from build123d import *

# Parameters (mm, degrees)
SKETCH1_W           = 22
SKETCH1_H           = 13
BOSS_EXTRUDE1_DEPTH = 6
BOSS_EXTRUDE2_DEPTH = 2
BOSS_EXTRUDE3_DEPTH = 8
SKETCH4_R           = 1.525
SKETCH4_R_2         = 1.524
CUT_EXTRUDE1_DEPTH  = 36.566838488
SKETCH5_W           = 9
SKETCH5_H           = 4.088652256
CUT_EXTRUDE2_DEPTH  = 38.735924528
FILLET1_R           = 2
SKETCH6_W           = 12
SKETCH6_H           = 13.009000019
SKETCH6_W_2         = 15.838286437
CUT_EXTRUDE3_DEPTH  = 4
SKETCH7_W           = 2.5
SKETCH7_H           = 8
BOSS_EXTRUDE5_DEPTH = 3
FILLET3_R           = 2.5
FILLET4_R           = 2.5
SKETCH9_W           = 24
SKETCH9_H           = 8
CUT_EXTRUDE5_DEPTH  = 3
BOSS_EXTRUDE6_REACH = 35.526
SKETCH10_W          = 5
SKETCH10_H          = 2.5
BOSS_EXTRUDE7_DEPTH = 2
SKETCH12_R          = 7.5
BOSS_EXTRUDE8_DEPTH = 8
SKETCH13_R          = 3.8735
CUT_EXTRUDE6_DEPTH  = 8
FILLET5_R           = 1.5
FILLET7_R           = 1


with BuildPart() as part:
    # Sketch1 → Boss-Extrude1 (new body)
    with BuildSketch(Plane(origin=(0, 0, 0), x_dir=(1, 0, 0), z_dir=(0, 1, 0))):
        with BuildLine():
            Line((-1, -3), (23, -3))
            Line((23, -3), (25, -3))
            Line((25, -3), (25, -1))
            Line((25, -1), (25, 14))
            Line((25, 14), (25, 16))
            Line((25, 16), (23, 16))
            Line((23, 16), (-1, 16))
            ThreePointArc((-1, 16), (-2.414213562, 15.414213562), (-3, 14))
            Line((-3, 14), (-3, -1))
            ThreePointArc((-3, -1), (-2.414213562, -2.414213562), (-1, -3))
        make_face()
        with Locations((11, 6.5)):
            Rectangle(SKETCH1_W, SKETCH1_H, mode=Mode.SUBTRACT)
    extrude(amount=BOSS_EXTRUDE1_DEPTH)

    # Sketch2 → Boss-Extrude2 (add)
    with BuildSketch(Plane(origin=(0, 6, 0), x_dir=(1, 0, 0), z_dir=(0, 1, 0))):
        with BuildLine():
            Line((25, 14), (25, -1))
            Line((25, -1), (25, -3))
            Line((25, -3), (23, -3))
            Line((23, -3), (-1, -3))
            ThreePointArc((-1, -3), (-2.414213562, -2.414213562), (-3, -1))
            Line((-3, -1), (-3, 14))
            ThreePointArc((-3, 14), (-2.414213562, 15.414213562), (-1, 16))
            Line((-1, 16), (23, 16))
            Line((23, 16), (25, 16))
            Line((25, 16), (25, 14))
        make_face()
    extrude(amount=BOSS_EXTRUDE2_DEPTH)

    # Sketch3 → Boss-Extrude3 (add)
    with BuildSketch(Plane.XZ):
        with BuildLine():
            Line((5, 3), (17, 3))
            Line((17, 3), (17, 5.5))
            ThreePointArc((17, 5.5), (15.389087297, 9.389087297), (11.5, 11))
            Line((11.5, 11), (10.5, 11))
            ThreePointArc((10.5, 11), (6.610912703, 9.389087297), (5, 5.5))
            Line((5, 5.5), (5, 3))
        make_face()
        with BuildLine():
            Line((17, -16), (5, -16))
            Line((5, -16), (5, -18.5))
            ThreePointArc((5, -18.5), (6.610912703, -22.389087297), (10.5, -24))
            Line((10.5, -24), (11.5, -24))
            ThreePointArc((11.5, -24), (15.389087297, -22.389087297), (17, -18.5))
            Line((17, -18.5), (17, -16))
        make_face()
    extrude(amount=-BOSS_EXTRUDE3_DEPTH)

    # Sketch4 → Cut-Extrude1 (cut, through all)
    with BuildSketch(Plane(origin=(0, 0, 0), x_dir=(-1, 0, 0), z_dir=(0, -1, 0))):
        with Locations(Location((-11, 20, 0), (0, 0, 90))):
            Circle(SKETCH4_R)
        with Locations(Location((-11, -7, 0), (0, 0, 90))):
            Circle(SKETCH4_R_2)
    extrude(amount=-CUT_EXTRUDE1_DEPTH, mode=Mode.SUBTRACT)

    # Sketch5 → Cut-Extrude2 (cut, through all)
    with BuildSketch(Plane(origin=(25, 0, 0), x_dir=(0, 0, -1), z_dir=(1, 0, 0))):
        with Locations((6.5, 2.044326128)):
            Rectangle(SKETCH5_W, SKETCH5_H)
    extrude(amount=-CUT_EXTRUDE2_DEPTH, mode=Mode.SUBTRACT)

    # Fillet1
    fillet1_edges = [part.edges().sort_by_distance(p)[0] for p in [
        (-1.5, 4.088652256, -11),
        (-1.5, 4.088652256, -2),
        (23.5, 4.088652256, -11),
        (23.5, 4.088652256, -2),
    ]]
    fillet(fillet1_edges, radius=FILLET1_R)

    # Sketch6 → Cut-Extrude3 (cut)
    with BuildSketch(Plane(origin=(0, 8, 0), x_dir=(1, 0, 0), z_dir=(0, 1, 0))):
        with Locations((11, 22.504500009)):
            Rectangle(SKETCH6_W, SKETCH6_H)
        with Locations((11.149066226, -9.50450001)):
            Rectangle(SKETCH6_W_2, SKETCH6_H)
    extrude(amount=-CUT_EXTRUDE3_DEPTH, mode=Mode.SUBTRACT)

    # Sketch7 → Boss-Extrude5 (add)
    with BuildSketch(Plane(origin=(25, 0, 0), x_dir=(0, 0, -1), z_dir=(1, 0, 0))):
        with Locations((17.25, 4)):
            Rectangle(SKETCH7_W, SKETCH7_H)
        with Locations((-4.25, 4)):
            Rectangle(SKETCH7_W, SKETCH7_H)
    extrude(amount=-BOSS_EXTRUDE5_DEPTH)

    # Fillet3
    fillet3_edges = [part.edges().sort_by_distance(p)[0] for p in [
        (22, 4, -16),
    ]]
    fillet(fillet3_edges, radius=FILLET3_R - 0.0001)  # a hair under: the kernel refuses the full size

    # Fillet4
    fillet4_edges = [part.edges().sort_by_distance(p)[0] for p in [
        (22, 4, 3),
    ]]
    fillet(fillet4_edges, radius=FILLET4_R - 0.0001)  # a hair under: the kernel refuses the full size

    # Sketch9 → Cut-Extrude5 (cut)
    with BuildSketch(Plane(origin=(25, 0, 0), x_dir=(0, 0, -1), z_dir=(1, 0, 0))):
        with Locations((6.5, 4)):
            Rectangle(SKETCH9_W, SKETCH9_H)
    extrude(amount=-CUT_EXTRUDE5_DEPTH, mode=Mode.SUBTRACT)

    # Boss-Extrude6: up to this face of the body (flat: up to its plane)
    boss_extrude6_end = Plane(part.part.faces().sort_by_distance((9.97036164, 0, 3.836684907))[0])
    # Sketch10 → Boss-Extrude6 (add, up to the picked face)
    with BuildSketch(Plane(origin=(0, 8, 0), x_dir=(1, 0, 0), z_dir=(0, 1, 0)), mode=Mode.PRIVATE) as boss_extrude6_sk1:
        with Locations((19.5, 17.25)):
            Rectangle(SKETCH10_W, SKETCH10_H)
    boss_extrude6_tool1 = split(extrude(boss_extrude6_sk1.sketch, amount=-BOSS_EXTRUDE6_REACH, mode=Mode.PRIVATE), bisect_by=boss_extrude6_end, keep=Keep.BOTH, mode=Mode.PRIVATE)
    # Sketch10 → Boss-Extrude6 (add, up to the picked face)
    with BuildSketch(Plane(origin=(0, 8, 0), x_dir=(1, 0, 0), z_dir=(0, 1, 0)), mode=Mode.PRIVATE) as boss_extrude6_sk2:
        with Locations((19.5, -4.25)):
            Rectangle(SKETCH10_W, SKETCH10_H)
    boss_extrude6_tool2 = split(extrude(boss_extrude6_sk2.sketch, amount=-BOSS_EXTRUDE6_REACH, mode=Mode.PRIVATE), bisect_by=boss_extrude6_end, keep=Keep.BOTH, mode=Mode.PRIVATE)
    add(boss_extrude6_tool1.solids().sort_by(Axis((19.5, 8, -17.25), (0, -1, 0)))[0])
    add(boss_extrude6_tool2.solids().sort_by(Axis((19.5, 8, 4.25), (0, -1, 0)))[0])

    # Sketch11 → Boss-Extrude7 (add)
    with BuildSketch(Plane(origin=(0, 8, 0), x_dir=(1, 0, 0), z_dir=(0, 1, 0))):
        with BuildLine():
            Line((17, -3), (-1, -3))
            ThreePointArc((-1, -3), (-2.414213562, -2.414213562), (-3, -1))
            Line((-3, -1), (-3, 14))
            ThreePointArc((-3, 14), (-2.414213562, 15.414213562), (-1, 16))
            Line((-1, 16), (17, 16))
            Line((17, 16), (17, 18.5))
            Line((17, 18.5), (22, 18.5))
            Line((22, 18.5), (22, -5.5))
            Line((22, -5.5), (17, -5.5))
            Line((17, -5.5), (17, -3))
        make_face()
    extrude(amount=BOSS_EXTRUDE7_DEPTH)

    # Sketch12 → Boss-Extrude8 (add)
    with BuildSketch(Plane(origin=(0, 10, 0), x_dir=(1, 0, 0), z_dir=(0, 1, 0))):
        with Locations(Location((9.5, 6.5, 0), (0, 0, 90))):
            Circle(SKETCH12_R)
    extrude(amount=BOSS_EXTRUDE8_DEPTH)

    # Sketch13 → Cut-Extrude6 (cut)
    with BuildSketch(Plane(origin=(0, 18, 0), x_dir=(1, 0, 0), z_dir=(0, 1, 0))):
        with Locations(Location((9.5, 6.5, 0), (0, 0, 270))):
            Circle(SKETCH13_R)
    extrude(amount=-CUT_EXTRUDE6_DEPTH, mode=Mode.SUBTRACT)

    # Fillet5
    fillet5_edges = [part.edges().sort_by_distance(p)[0] for p in [
        (9.5, 10, 1),
    ]]
    fillet(fillet5_edges, radius=FILLET5_R)

    # Fillet7
    fillet7_edges = [part.edges().sort_by_distance(p)[0] for p in [
        (9.5, 18, 1),
    ]]
    fillet(fillet7_edges, radius=FILLET7_R)


solid = part.part
Here's how the part is built. I have some questions about the finished solid (model axes, mm). A direction names the side the tool comes from. Round coordinates to 2 decimals unless told otherwise and drop trailing zeros. Write each loop counter-clockwise with the first axis right and the second up, starting at its lowest first coordinate (ties: lowest second). Pieces come first, ordered by that corner, then holes. Notation, with made-up numbers: (41.5, 42) -> (89.5, 42) arc R9 ccw to (89.5, 57) -> close; hole circle Ø10 at (-0.75, 12). An arc over 180 degrees is marked (long way). One line per item, written item: value.
1) Suppose I cut it at D-D on x = -1.5. List the corners of the cut face in (y, z) for me, plus the area to 3 significant figures.
Filled sheet:
outline: (0, -15.94) -> (10, -15.94) -> (10, 2.94) -> (0, 2.94) -> (0, -2) -> (2.09, -2) arc R2 cw to (4.09, -4) -> (4.09, -9) arc R2 cw to (2.09, -11) -> (0, -11) -> close
area: 154 mm2
2) Suppose I cut it at A-A on z = -20. List the corners of the cut face in (x, y) for me (1 decimal).
Filled sheet:
outline: (5.2, 0) -> (9.5, 0) -> (9.5, 4) -> (5.2, 4) -> close; (12.5, 0) -> (16.8, 0) -> (16.8, 4) -> (12.5, 4) -> close
3) For faces 1 (the face through (-1, 1, -11)), 2 (the face through (13.34, 14.06, -7)), 3 (the face through (5, 2, 4)), which set-ups out of +Z, -Z, +X, -X, +Y, -Y let a thin tool reach every point of the face, with its end or its side?
Filled sheet:
face 1: +X, -X, -Y
face 2: +Y
face 3: +Z, -X, +Y, -Y
4) I'm going to push flat-ended pins straight in: pin 1 Ø3 at (x, y) = (15.5, 13.5) entering from +Z; pin 2 Ø5.5 at (x, y) = (19, 4) entering from -Z; pin 3 Ø5 at (x, y) = (14.5, 3) entering from -Z. Where does each tip first touch, or does it pass through?
Filled sheet:
pin 1: stops at z = -0.5
pin 2: stops at z = -21.27
pin 3: stops at z = -23.98
5) Suppose I cut it at B-B on y = 3.5. List the corners of the cut face in (x, z) for me (3 decimals), plus the area to 3 significant figures.
Filled sheet:
outline: (-3, -14) arc R2 ccw to (-1, -16) -> (5, -16) -> (5, -18.5) arc R5.5 ccw to (10.5, -24) -> (11.5, -24) arc R5.5 ccw to (17, -18.5) -> (22, -18.5) -> (22, -13) -> (0, -13) -> (0, -10.417) -> (-3, -10.417) -> close; (-3, -2.583) -> (0, -2.583) -> (0, 0) -> (22, 0) -> (22, 5.5) -> (17, 5.5) arc R5.5 ccw to (11.5, 11) -> (10.5, 11) arc R5.5 ccw to (5, 5.5) -> (5, 3) -> (-1, 3) arc R2 ccw to (-3, 1) -> close; hole circle Ø3.05 at (11, -20); hole circle Ø3.048 at (11, 7)
area: 340 mm2
6) If I drill on line 1 (Z direction, x = 9.25, y = 5.75); line 2 (Y direction, x = 17.5, z = -18); line 3 (Z direction, x = 2.5, y = 9.75), over which ranges is the centre line in solid material (lowest first)? Write a range as [from, to].
Filled sheet:
line 1: z = [-16, -13], [0, 3]
line 2: y = [0, 10]
line 3: z = [-16, 3]
7) Suppose I cut it at C-C on z = 4. List the corners of the cut face in (x, y) for me.
Filled sheet:
outline: (5, 0) -> (22, 0) -> (22, 10) -> (17, 10) -> (17, 4) -> (5, 4) -> close
8) We'd pull the mould along Z, two halves only. Please class faces 4 (the face through (15.35, 1.97, -22.43)), 5 (the face through (11, 3, -13)), 6 (the face through (17, 7, -17)): released by +Z, released by -Z, zero draft, split by the parting line, or undercut.
Filled sheet:
face 4: released by -Z
face 5: undercut
face 6: zero draft
